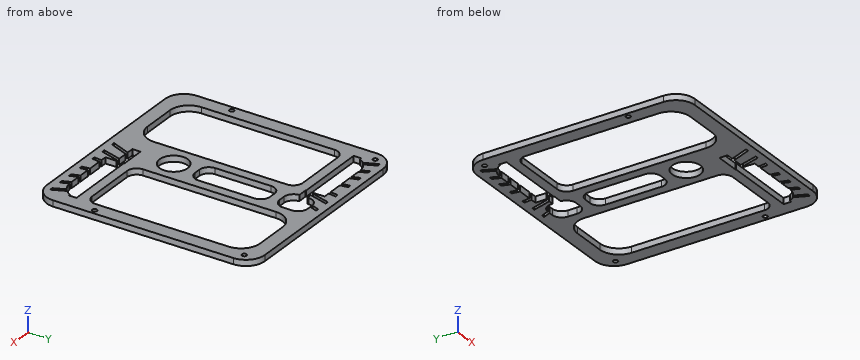
from build123d import *

# Parameters (mm, degrees)
SKETCH1_W           = 57.8674
SKETCH1_H           = 58.2902
SKETCH1_W_2         = 50.2474
SKETCH1_H_2         = 50.6702
BOSS_EXTRUDE1_DEPTH = 1.5875
FILLET3_R           = 5.08
SKETCH6_W           = 11.8934
SKETCH6_H           = 50.6702
SKETCH6_R           = 3.7592
BOSS_EXTRUDE2_DEPTH = 1.5875
FINS_CUT_DEPTH      = 2.54
SKETCH7_W           = 19.177
SKETCH7_H           = 2.54
BOSS_EXTRUDE3_DEPTH = 1.5875
FILLET1_R           = 5.08
FILLET4_R           = 5.08
SKETCH8_W           = 6.8134
SKETCH8_H           = 7.493
SKETCH8_H_2         = 20.0392
CUT_EXTRUDE5_DEPTH  = 1.5875
FILLET5_R           = 2.54
FILLET6_R           = 2.54
FILLET7_R           = 2.54
SKETCH9_R           = 0.6096
CUT_EXTRUDE6_DEPTH  = 1.5875


with BuildPart() as part:
    # Sketch1 → Boss-Extrude1 (new body)
    with BuildSketch(Plane.XY):
        with Locations((12.492699517, 17.740517652)):
            Rectangle(SKETCH1_W, SKETCH1_H)
        with Locations((12.492699517, 17.740517652)):
            Rectangle(SKETCH1_W_2, SKETCH1_H_2, mode=Mode.SUBTRACT)
    extrude(amount=BOSS_EXTRUDE1_DEPTH)

    # Fillet3
    fillet3_edges = [part.edges().sort_by_distance(p)[0] for p in [
        (-12.631000483, 43.075617652, 0.79375),
        (-12.631000483, -7.594582348, 0.79375),
        (37.616399517, -7.594582348, 0.79375),
        (37.616399517, 43.075617652, 0.79375),
    ]]
    fillet(fillet3_edges, radius=FILLET3_R)

    # Sketch6 → Boss-Extrude2 (add)
    with BuildSketch(Plane.XY.offset(1.5875)):
        with Locations((12.492699517, 17.740517652)):
            Rectangle(SKETCH6_W, SKETCH6_H)
        with Locations((12.492699517, 6.704217652)):
            Circle(SKETCH6_R, mode=Mode.SUBTRACT)
    extrude(amount=-BOSS_EXTRUDE2_DEPTH)

    # Sketch4 → Fins cut (cut)
    with BuildSketch(Plane.XY.offset(1.5875)):
        with BuildLine():
            Line((-12.149382698, 40.154617652), (-12.631000483, 40.154617652))
            Line((-12.631000483, 40.154617652), (-12.631000483, 37.995617652))
            ThreePointArc((-12.631000483, 37.995617652), (-12.509134288, 39.101650731), (-12.149382698, 40.154617652))
        make_face()
        Polygon((6.545999517, 40.154617652), (6.545999517, 37.995617652), (13.022999517, 37.995617652), (13.022999517, 40.154617652), (11.126956513, 40.154617652), (13.082688495, 45.107617652), (12.263436468, 45.107617652), (10.307704486, 40.154617652), (7.705138754, 40.154617652), (9.127606772, 45.107617652), (8.317171321, 45.107617652), (6.894703303, 40.154617652), align=None)
        with BuildLine():
            Line((-12.701104011, 45.107617652), (-11.115909096, 41.614709607))
            ThreePointArc((-11.115909096, 41.614709607), (-10.827291356, 41.877926001), (-10.5193022, 42.118187835))
            Line((-10.5193022, 42.118187835), (-11.876002372, 45.107617652))
            Line((-11.876002372, 45.107617652), (-12.701104011, 45.107617652))
        make_face()
        Polygon((4.93970469, 43.075617652), (5.163773621, 45.107617652), (4.362066012, 45.107617652), (4.137997081, 43.075617652), align=None)
        Polygon((18.439399517, -2.514582348), (11.962399517, -2.514582348), (11.962399517, -4.673582348), (13.858442521, -4.673582348), (11.902710539, -9.626582348), (12.721962566, -9.626582348), (14.677694548, -4.673582348), (17.28026028, -4.673582348), (15.857792262, -9.626582348), (16.668227713, -9.626582348), (18.090695731, -4.673582348), (18.439399517, -4.673582348), align=None)
        with BuildLine():
            Line((-8.755473368, 45.107617652), (-7.926673781, 43.061707818))
            ThreePointArc((-7.926673781, 43.061707818), (-7.738965845, 43.072139003), (-7.551000483, 43.075617652))
            Line((-7.551000483, 43.075617652), (-7.112090465, 43.075617652))
            Line((-7.112090465, 43.075617652), (-7.935255168, 45.107617652))
            Line((-7.935255168, 45.107617652), (-8.755473368, 45.107617652))
        make_face()
        with BuildLine():
            Line((37.616399517, -4.673582348), (37.616399517, -2.514582348))
            ThreePointArc((37.616399517, -2.514582348), (37.494533322, -3.620615427), (37.134781733, -4.673582348))
            Line((37.134781733, -4.673582348), (37.616399517, -4.673582348))
        make_face()
        Polygon((0.346695583, 43.075617652), (0.065397546, 45.107617652), (-0.737192749, 45.107617652), (-0.455894712, 43.075617652), align=None)
        with BuildLine():
            Line((37.686503045, -9.626582348), (36.10130813, -6.133674303))
            ThreePointArc((36.10130813, -6.133674303), (35.81269039, -6.396890696), (35.504701234, -6.637152531))
            Line((35.504701234, -6.637152531), (36.861401406, -9.626582348))
            Line((36.861401406, -9.626582348), (37.686503045, -9.626582348))
        make_face()
        Polygon((20.045694344, -7.594582348), (19.821625413, -9.626582348), (20.623333022, -9.626582348), (20.847401953, -7.594582348), align=None)
        Polygon((-5.00684021, 45.107617652), (-4.360824225, 43.075617652), (-3.54812875, 43.075617652), (-4.194144736, 45.107617652), align=None)
        Polygon((24.638703451, -7.594582348), (24.920001488, -9.626582348), (25.722591783, -9.626582348), (25.441293746, -7.594582348), align=None)
        with BuildLine():
            Line((33.740872402, -9.626582348), (32.912072815, -7.580672514))
            ThreePointArc((32.912072815, -7.580672514), (32.72436488, -7.591103698), (32.536399517, -7.594582348))
            Line((32.536399517, -7.594582348), (32.097489499, -7.594582348))
            Line((32.097489499, -7.594582348), (32.920654202, -9.626582348))
            Line((32.920654202, -9.626582348), (33.740872402, -9.626582348))
        make_face()
        Polygon((28.533527785, -7.594582348), (29.17954377, -9.626582348), (29.992239244, -9.626582348), (29.346223259, -7.594582348), align=None)
    extrude(amount=-FINS_CUT_DEPTH, mode=Mode.SUBTRACT)

    # Sketch7 → Boss-Extrude3 (add)
    with BuildSketch(Plane.XY.offset(1.5875)):
        with Locations((-3.042500483, 36.852617652)):
            Rectangle(SKETCH7_W, SKETCH7_H)
        with Locations((28.027899517, -1.371582348)):
            Rectangle(SKETCH7_W, SKETCH7_H)
    extrude(amount=-BOSS_EXTRUDE3_DEPTH)

    # Fillet1
    fillet1_edges = [part.edges().sort_by_distance(p)[0] for p in [
        (-16.441000483, 46.885617652, 0.79375),
        (41.426399517, 46.885617652, 0.79375),
        (41.426399517, -11.404582348, 0.79375),
        (-16.441000483, -11.404582348, 0.79375),
    ]]
    fillet(fillet1_edges, radius=FILLET1_R)

    # Fillet4
    fillet4_edges = [part.edges().sort_by_distance(p)[0] for p in [
        (6.545999517, -7.594582348, 0.79375),
        (18.439399517, 43.075617652, 0.79375),
    ]]
    fillet(fillet4_edges, radius=FILLET4_R)

    # Sketch8 → Cut-Extrude5 (cut)
    with BuildSketch(Plane.XY.offset(1.5875)):
        with Locations((12.492699517, 39.329117652)):
            Rectangle(SKETCH8_W, SKETCH8_H)
        with Locations((12.492699517, 23.023017652)):
            Rectangle(SKETCH8_W, SKETCH8_H_2)
    extrude(amount=-CUT_EXTRUDE5_DEPTH, mode=Mode.SUBTRACT)

    # Fillet5
    # the kernel refuses this fillet: 2.54 mm, written as the material it adds along each edge
    with BuildSketch(Plane(origin=(9.085999517, 43.075617652, 1.5875), x_dir=(1, 0, 0), z_dir=(0, 0, -1))) as fillet5_piece_1:
        with BuildLine():
            CenterArc((2.54, 2.534640638), FILLET5_R, 180, 86.277337152)
            Line((0, 2.534640638), (-0.0508, 2.534640638))
            Line((-0.0508, 2.534640638), (-0.0508, 0))
            Line((-0.0508, 0), (0, -0.0508))
            ThreePointArc((0, -0.0508), (1.187542685, -0.0508), (2.371787076, -0.050692813))
            Line((2.371787076, -0.050692813), (2.375085369, 0))
        make_face()
    extrude(amount=1.5875)
    with BuildSketch(Plane(origin=(15.899399517, 43.075617652, 1.5875), x_dir=(0, -1, 0), z_dir=(0, 0, -1)), Plane(origin=(9.085999517, 13.003417652, 1.5875), x_dir=(0, 1, 0), z_dir=(0, 0, -1)), Plane(origin=(15.899399517, 13.003417652, 1.5875), x_dir=(-1, 0, 0), z_dir=(0, 0, -1))) as fillet5_piece_2:
        with BuildLine():
            CenterArc((FILLET5_R, FILLET5_R), FILLET5_R, 180, 90)
            Line((0, FILLET5_R), (-FILLET5_R * 0.02, FILLET5_R))
            Line((-FILLET5_R * 0.02, FILLET5_R), (-FILLET5_R * 0.02, -FILLET5_R * 0.02))
            Line((-FILLET5_R * 0.02, -FILLET5_R * 0.02), (FILLET5_R, -FILLET5_R * 0.02))
            Line((FILLET5_R, -FILLET5_R * 0.02), (FILLET5_R, 0))
        make_face()
    extrude(amount=1.5875)

    # Fillet6
    fillet6_edges = [part.edges().sort_by_distance(p)[0] for p in [
        (6.545999517, 35.582617652, 0.79375),
        (-12.631000483, 35.582617652, 0.79375),
        (18.439399517, -0.101582348, 0.79375),
        (37.616399517, -0.101582348, 0.79375),
    ]]
    fillet(fillet6_edges, radius=FILLET6_R)

    # Fillet7
    # the kernel refuses this fillet: 2.54 mm, written as the material it adds along each edge
    with BuildSketch(Plane(origin=(9.085999517, 35.582617652, 1.5875), x_dir=(1, 0, 0), z_dir=(0, 0, -1))) as fillet7_piece_1:
        with BuildLine():
            CenterArc((2.536823013, -2.54), FILLET7_R, 90, 87.134016017)
            Line((0, -2.413), (-0.05073646, -2.41046))
            ThreePointArc((-0.05073646, -2.41046), (-0.0508, -1.2065), (-0.0508, 0))
            Line((-0.0508, 0), (0, 0.0508))
            Line((0, 0.0508), (2.536823013, 0.0508))
            Line((2.536823013, 0.0508), (2.536823013, 0))
        make_face()
    extrude(amount=1.5875)
    with BuildSketch(Plane(origin=(15.899399517, 35.582617652, 1.5875), x_dir=(0, 1, 0), z_dir=(0, 0, -1)), Plane(origin=(15.899399517, 33.042617652, 1.5875), x_dir=(-1, 0, 0), z_dir=(0, 0, -1))) as fillet7_piece_2:
        with BuildLine():
            CenterArc((FILLET7_R, -FILLET7_R), FILLET7_R, 90, 90)
            Line((0, -FILLET7_R), (-FILLET7_R * 0.02, -FILLET7_R))
            Line((-FILLET7_R * 0.02, -FILLET7_R), (-FILLET7_R * 0.02, FILLET7_R * 0.02))
            Line((-FILLET7_R * 0.02, FILLET7_R * 0.02), (FILLET7_R, FILLET7_R * 0.02))
            Line((FILLET7_R, FILLET7_R * 0.02), (FILLET7_R, 0))
        make_face()
    extrude(amount=1.5875)
    with BuildSketch(Plane(origin=(9.085999517, 33.042617652, 1.5875), x_dir=(1, 0, 0), z_dir=(0, 0, -1))) as fillet7_piece_3:
        with BuildLine():
            CenterArc((FILLET7_R, FILLET7_R), FILLET7_R, 180, 90)
            Line((0, FILLET7_R), (-FILLET7_R * 0.02, FILLET7_R))
            Line((-FILLET7_R * 0.02, FILLET7_R), (-FILLET7_R * 0.02, -FILLET7_R * 0.02))
            Line((-FILLET7_R * 0.02, -FILLET7_R * 0.02), (FILLET7_R, -FILLET7_R * 0.02))
            Line((FILLET7_R, -FILLET7_R * 0.02), (FILLET7_R, 0))
        make_face()
    extrude(amount=1.5875)

    # Sketch9 → Cut-Extrude6 (cut)
    with BuildSketch(Plane.XY.offset(1.5875)):
        with Locations((-13.901000483, 43.075617652)):
            Circle(SKETCH9_R)
        with Locations((38.886399517, 43.075617652)):
            Circle(SKETCH9_R)
        with Locations((40.130999517, 3.910217652)):
            Circle(SKETCH9_R)
        with Locations((-15.145600483, 3.910217652)):
            Circle(SKETCH9_R)
    extrude(amount=-CUT_EXTRUDE6_DEPTH, mode=Mode.SUBTRACT)


solid = part.part
Input: part model. Units: mm. Frame: model coordinates. Round coordinates to 2 decimals unless told otherwise and drop trailing zeros. Loops run counter-clockwise (first coordinate to the right, second up) from the corner with the lowest first, then second, coordinate; pieces in that order, holes last. Notation, with made-up numbers: (8, -9.75) -> (44, -9.75) arc R23 ccw to (44, 5.25) -> close; hole circle Ø1 at (-30, 19.5). An arc over 180 degrees is marked (long way). Answer as a JSON object with one key per item and string values. Group by question number.
1) Ray query, L1, parallel to Y at x = -3.5, z = 0.95; L2, parallel to X at y = 30, z = 0.4; L3, parallel to Y at x = 26, z = 0.5. Return the intervals inside material, ascending.
2) Pin query (flat end, axial travel): pin 1 (1.6 mm diameter, centred on x = -13.9, y = 43.08, fed in from +Z). Return the tip coordinate at first contact, or that it passes through.
3) Section query A-A on y = -1. Output: boundary loops of the cut face in (x, z).
4) Section query C-C on z = 0.45. State how many separate pieces and enclosed holes the cut face has, plus the area to 3 significant figures.
5) Section query B-B on y = 37. Output: boundary loops of the cut face in (x, z), plus the area to 3 significant figures.
Reply:
{
 "1": {"L1": "y = -11.4 to -7.59, 35.58 to 38.12, 43.08 to 46.89", "L2": "x = -16.44 to -12.63, 6.55 to 9.09, 15.9 to 18.44, 37.62 to 41.43", "L3": "y = -11.4 to -7.59, -2.64 to -0.1, 43.08 to 46.89"},
 "2": {"pin 1": "stops at z = 1.59"},
 "3": {"outline": "(-16.44, 0) -> (-12.63, 0) -> (-12.63, 1.59) -> (-16.44, 1.59) -> close; (6.55, 0) -> (41.43, 0) -> (41.43, 1.59) -> (6.55, 1.59) -> close"},
 "4": {"separate pieces": "1", "enclosed holes": "10", "area": "1,270 mm2"},
 "5": {"outline": "(-16.44, 0) -> (9.34, 0) -> (9.34, 1.59) -> (-16.44, 1.59) -> close; (15.64, 0) -> (18.44, 0) -> (18.44, 1.59) -> (15.64, 1.59) -> close; (37.62, 0) -> (41.43, 0) -> (41.43, 1.59) -> (37.62, 1.59) -> close", "area": "51.4 mm2"}
}
